Design review of the part built by this model. Coordinates are the model's own, in mm. Face numbers are marked on the shaded views. A direction names the side the tool comes from. Coordinates: 2 decimals unless noted, no trailing zeros. Loops run counter-clockwise (first coordinate to the right, second up) from the corner with the lowest first, then second, coordinate; pieces in that order, holes last.
Q1. Machinability: for the marked faces 1, 2 and 3, which of the approach directions +Z, -Z, +X, -X, +Y, -Y give a long, thin tool a straight path to every point of the face, cutting with its end or side? Answer none if there is none.
Q2. Add section D-D on z = 0.75. Give the boundary of the cut face in (x, y), and give its area (3 significant figures).
Q3. Wall thickness on probe 1 along Y at (x, z) = (0, 0.3); probe 2 along Y at (x, z) = (0, -1.5); probe 3 along Z at (x, y) = (4, -2): over which ranges is each line inside the solid? List them lowest first.
Q4. For P1, Ø5, axis at x = -5, z = 4, coming from the -Y side; P2, Ø3, axis at x = 0, y = 0, coming from the +Z side; P3, Ø6, axis at x = -6.5, z = 4.5, coming from the -Y side; P4, Ø6, axis at x = -3.5, y = -3.5, coming from the +Z side, all flat-tipped, find the tip position at first contact; note any pin that passes through.
Q5. Add section A-A on z = 6. Give the boundary of the cut face in (x, y).
Q6. Add section B-B on y = 0. Give the boundary of the cut face in (x, z), and give its area (3 significant figures).
Q7. Draft analysis for pull direction Y (two halves, no side actions). For the marked faces 4, 5 and 6, state which applies: released by +Y, released by -Y, zero draft, split by the parting line, or undercut.
Q8. Add section C-C on x = 0. Give the boundary of the cut face in (y, z), and give its area (3 significant figures).
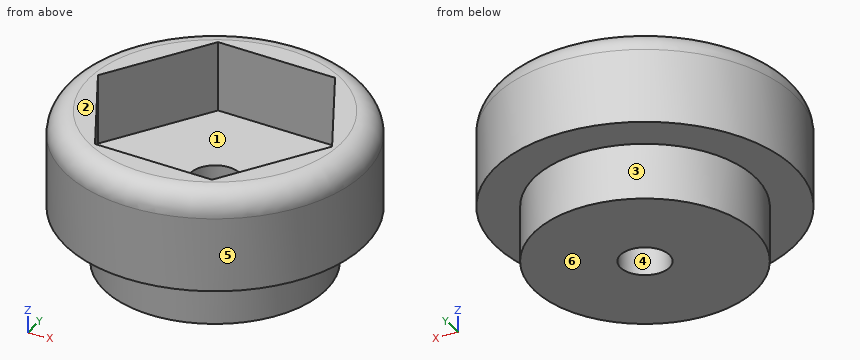
```python
from build123d import *
from build123d import SkipClean  # not in build123d's __all__

# Parameters (mm, degrees)
F0_R      = 10.668
F1_DEPTH  = 7
F4_DEPTH  = 2
F7_DEPTH  = 2
F8_R      = 7.8995
F9_DEPTH  = 6
F5_R      = 1.75
F10_DEPTH = 25
F11_R     = 1.7


with BuildPart() as f1:
    # F0 (on Top) → F1 (new body)
    with BuildSketch(Plane.XY):
        Circle(F0_R)
        Polygon((-4.8043411611, -7.2054358652), (-8.6422610852, 0.5579635614), (-3.837919924, 7.7633994266), (4.8043411611, 7.2054358652), (8.6422610852, -0.5579635614), (3.837919924, -7.7633994266), align=None, mode=Mode.SUBTRACT)
    extrude(amount=F1_DEPTH)

    # F3 (on offset) → F4 (join)
    with BuildSketch(Plane(origin=(0, 0, 2), x_dir=(1, 0, 0), z_dir=(0, 0, -1))):
        with BuildLine():
            ThreePointArc((1.9919788729, 7.6442213744), (3.5007804976, 7.081428963), (4.8641016704, 6.2243566085))
            Line((4.8641016704, 6.2243566085), (3.837919924, 7.7633994266))
            Line((3.837919924, 7.7633994266), (1.9919788729, 7.6442213744))
        make_face()
        with BuildLine():
            ThreePointArc((-5.6241004659, 5.5472149949), (-4.3823071282, 6.5724793255), (-2.95840011, 7.3246139174))
            Line((-2.95840011, 7.3246139174), (-4.8043411611, 7.2054358652))
            Line((-4.8043411611, 7.2054358652), (-5.6241004659, 5.5472149949))
        make_face()
        with BuildLine():
            ThreePointArc((-7.6160793388, -2.0970063795), (-7.8830876258, -0.5089496375), (-7.8225017804, 1.1002573089))
            Line((-7.8225017804, 1.1002573089), (-8.6422610852, -0.5579635614))
            Line((-8.6422610852, -0.5579635614), (-7.6160793388, -2.0970063795))
        make_face()
        with BuildLine():
            Line((-3.837919924, -7.7633994266), (-1.9919788729, -7.6442213744))
            ThreePointArc((-1.9919788729, -7.6442213744), (-3.5007804976, -7.081428963), (-4.8641016704, -6.2243566085))
            Line((-4.8641016704, -6.2243566085), (-3.837919924, -7.7633994266))
        make_face()
        with BuildLine():
            ThreePointArc((7.6160793388, 2.0970063795), (7.8283241817, 1.0580362738), (7.8995, 0))
            ThreePointArc((7.8995, 0), (7.880226934, -0.5514741317), (7.8225017804, -1.1002573089))
            Line((7.8225017804, -1.1002573089), (8.6422610852, 0.5579635614))
            Line((8.6422610852, 0.5579635614), (7.6160793388, 2.0970063795))
        make_face()
        with BuildLine():
            Line((4.8043411611, -7.2054358652), (5.6241004659, -5.5472149949))
            ThreePointArc((5.6241004659, -5.5472149949), (4.3823071282, -6.5724793255), (2.95840011, -7.3246139174))
            Line((2.95840011, -7.3246139174), (4.8043411611, -7.2054358652))
        make_face()
    extrude(amount=F4_DEPTH)

    # F6 (on face) → F7 (cut)
    with BuildSketch(Plane(origin=(0, 0, 0), x_dir=(1, 0, 0), z_dir=(0, 0, -1))):
        with BuildLine():
            Line((4.8641016704, 6.2243566085), (7.6160793388, 2.0970063795))
            ThreePointArc((7.6160793388, 2.0970063795), (6.5724793255, 4.3823071282), (4.8641016704, 6.2243566085))
        make_face()
        with BuildLine():
            ThreePointArc((5.6241004659, -5.5472149949), (7.081428963, -3.5007804976), (7.8225017804, -1.1002573089))
            Line((7.8225017804, -1.1002573089), (5.6241004659, -5.5472149949))
        make_face()
        with BuildLine():
            ThreePointArc((-1.9919788729, -7.6442213744), (0.5089496375, -7.8830876258), (2.95840011, -7.3246139174))
            Line((2.95840011, -7.3246139174), (-1.9919788729, -7.6442213744))
        make_face()
        with BuildLine():
            ThreePointArc((-7.6160793388, -2.0970063795), (-6.5724793255, -4.3823071282), (-4.8641016704, -6.2243566085))
            Line((-4.8641016704, -6.2243566085), (-7.6160793388, -2.0970063795))
        make_face()
        with BuildLine():
            Line((-7.8225017804, 1.1002573089), (-5.6241004659, 5.5472149949))
            ThreePointArc((-5.6241004659, 5.5472149949), (-7.081428963, 3.5007804976), (-7.8225017804, 1.1002573089))
        make_face()
        with BuildLine():
            Line((-2.95840011, 7.3246139174), (1.9919788729, 7.6442213744))
            ThreePointArc((1.9919788729, 7.6442213744), (-0.5089496375, 7.8830876258), (-2.95840011, 7.3246139174))
        make_face()
    with SkipClean():  # cleaning this boolean's faces spoils the solid; the shape is the same uncleaned
        extrude(amount=-F7_DEPTH, mode=Mode.SUBTRACT)

    # F8 (on offset) → F9 (join)
    with BuildSketch(Plane(origin=(0, 0, 2), x_dir=(1, 0, 0), z_dir=(0, 0, -1))):
        Circle(F8_R)
    extrude(amount=F9_DEPTH)

    # F5 (on face) → F10 (cut)
    with BuildSketch(Plane.XY.offset(2)):
        Circle(F5_R)
    extrude(amount=-F10_DEPTH, mode=Mode.SUBTRACT)

    # F11
    f11_edges = [f1.edges().sort_by_distance(p)[0] for p in [
        (-10.668, 0, 7),
    ]]
    fillet(f11_edges, radius=F11_R)


solid = f1.part
```
Entries:
1. face 1: +Z
1. face 2: +Z, +X, -X, +Y, -Y
1. face 3: -Z
2. outline: circle Ø21.34 at (0, 0); hole circle Ø3.5 at (0, 0)
2. area: 348 mm2
3. probe 1: y = -10.67 to -1.75, 1.75 to 10.67
3. probe 2: y = -7.9 to -1.75, 1.75 to 7.9
3. probe 3: z = -4 to 2
4. P1: stops at y = -10.37
4. P2: passes through
4. P3: stops at y = -10.08
4. P4: stops at z = 7
5. outline: circle Ø21.03 at (0, 0); hole (-8.64, 0.56) - (-4.8, -7.21) - (3.84, -7.76) - (8.64, -0.56) - (4.8, 7.21) - (-3.84, 7.76) - close
6. outline: (-10.67, 0) - (-7.9, 0) - (-7.9, -4) - (-1.75, -4) - (-1.75, 2) - (-8.37, 2) - (-8.37, 7) - (-8.97, 7) arc R1.7 ccw to (-10.67, 5.3) - close; (1.75, -4) - (7.9, -4) - (7.9, 0) - (10.67, 0) - (10.67, 5.3) arc R1.7 ccw to (8.97, 7) - (8.37, 7) - (8.37, 2) - (1.75, 2) - close
6. area: 107 mm2
7. face 4: undercut
7. face 5: split by the parting line
7. face 6: zero draft
8. outline: (-10.67, 0) - (-7.9, 0) - (-7.9, -4) - (-1.75, -4) - (-1.75, 2) - (-7.52, 2) - (-7.52, 7) - (-8.97, 7) arc R1.7 ccw to (-10.67, 5.3) - close; (1.75, -4) - (7.9, -4) - (7.9, 0) - (10.67, 0) - (10.67, 5.3) arc R1.7 ccw to (8.97, 7) - (7.52, 7) - (7.52, 2) - (1.75, 2) - close
8. area: 115 mm2
